Geometry: final body of the model. Coordinates: model frame, mm. A direction names the side the tool comes from. Give positions to 0.01 mm unless a question says otherwise; leave off trailing zeros. Write each loop counter-clockwise with the first axis right and the second up, starting at its lowest first coordinate (ties: lowest second). Pieces come first, ordered by that corner, then holes. Notation, with made-up numbers: (-3, -4) -> (14, -4) arc R23 cw to (14, 24) -> close; hole circle Ø2 at (60, 57.25). An arc over 180 degrees is marked (long way). Use CSV: the item, a comma, the result in double quotes. Start each with the question number.
1) Section D-D (y = 1). Count the separate pieces of the cut face and the enclosed holes in it, plus the area to 3 significant figures.
2) Material intervals for line 1 (Z direction, x = -110.72, y = 1.15); line 2 (Z direction, x = 65, y = 0.3); line 3 (X direction, y = 0.95, z = -155), sorted ascending. Write a range as [from, to].
3) Section A-A (x = 148). Output: boundary loops of the cut face in (y, z).
4) Set-up query: faces 1 (the face through (-2, 0, -2)), 2 (the face through (-62.018, 0.74, -149.464)). Return all of +Z, -Z, +X, -X, +Y, -Y with unobstructed straight access to the full face (end or side cutting, diameter ignored); none if empty.
5) Section B-B (z = 80). Output: boundary loops of the cut face in (x, y), plus the area to 3 significant figures.
6) Contact query for flat-ended pins moving along their axis: P1, Ø3, axis at x = 65, z = 118.58, coming from the -Y side; P2, Ø0.8, axis at x = -135.5, y = 1, coming from the -Z side. Output: stop coordinate, or through.
7) Draft query along X for faces 3 (the face through (-150, 1, -150)), 4 (the face through (150, 1, 150)), 5 (the face through (-1.35, 0.74, 122.74)). Return one class per face: pulls with the +X half, pulls with the -X half, needs draft (parallel to the pull), parting line crosses it, or undercut.
8) Section C-C (z = 148). Output: boundary loops of the cut face in (x, y).
```python
from build123d import *

# Parameters (mm, degrees)
SKETCH_1_R          = 1.55
SKETCH_1_W          = 30.4
SKETCH_1_H          = 68.58
EXTRUDE_1_DEPTH     = 1.5
FILLET_1_R          = 10
FILLET_2_R          = 10
FILLET_3_R          = 10
SKETCH_1_5_R        = 2.05
CUT_EXTRUDE_3_DEPTH = 10


with BuildPart() as part:
    # 草图1 → 凸台-拉伸1 (new body)
    with BuildSketch(Plane(origin=(0, 0, 0), x_dir=(1, 0, 0), z_dir=(0, 1, 0))):
        with BuildLine():
            Line((-125, 175), (-175, 125))
            Line((-175, 125), (-175, -125))
            Line((-175, -125), (-125, -175))
            Line((-125, -175), (-81.710313025, -175))
            ThreePointArc((-81.710313025, -175), (0, -122.728301649), (81.710313025, -175))
            Line((81.710313025, -175), (125, -175))
            Line((125, -175), (175, -125))
            Line((175, -125), (175, 125))
            Line((175, 125), (125, 175))
            Line((125, 175), (85, 175))
            Line((85, 175), (40, 125))
            Line((40, 125), (40, 85))
            Line((40, 85), (-40, 85))
            Line((-40, 85), (-40, 125))
            Line((-40, 125), (-85, 175))
            Line((-85, 175), (-125, 175))
        make_face()
        with Locations((-55, 131)):
            Circle(SKETCH_1_R, mode=Mode.SUBTRACT)
        with Locations((-80, 160)):
            Circle(SKETCH_1_R, mode=Mode.SUBTRACT)
        with Locations((55, 131)):
            Circle(SKETCH_1_R, mode=Mode.SUBTRACT)
        with Locations((80, 160)):
            Circle(SKETCH_1_R, mode=Mode.SUBTRACT)
        with Locations((-65, 118.58)):
            Circle(SKETCH_1_R, mode=Mode.SUBTRACT)
        with Locations((-65, 50)):
            Circle(SKETCH_1_R, mode=Mode.SUBTRACT)
        with Locations((-110.72, 50)):
            Circle(SKETCH_1_R, mode=Mode.SUBTRACT)
        with Locations((-110.72, 118.58)):
            Circle(SKETCH_1_R, mode=Mode.SUBTRACT)
        with Locations((-164.434, 118.58)):
            Circle(SKETCH_1_R, mode=Mode.SUBTRACT)
        with Locations((-164.434, 50)):
            Circle(SKETCH_1_R, mode=Mode.SUBTRACT)
        with Locations((-65, -118.58)):
            Circle(SKETCH_1_R, mode=Mode.SUBTRACT)
        with Locations((-65, -50)):
            Circle(SKETCH_1_R, mode=Mode.SUBTRACT)
        with Locations((-110.72, -50)):
            Circle(SKETCH_1_R, mode=Mode.SUBTRACT)
        with Locations((-110.72, -118.58)):
            Circle(SKETCH_1_R, mode=Mode.SUBTRACT)
        with Locations((-164.434, -50)):
            Circle(SKETCH_1_R, mode=Mode.SUBTRACT)
        with Locations((-164.434, -118.58)):
            Circle(SKETCH_1_R, mode=Mode.SUBTRACT)
        with Locations((65, 50)):
            Circle(SKETCH_1_R, mode=Mode.SUBTRACT)
        with Locations((110.72, 50)):
            Circle(SKETCH_1_R, mode=Mode.SUBTRACT)
        with Locations((110.72, 118.58)):
            Circle(SKETCH_1_R, mode=Mode.SUBTRACT)
        with Locations((65, 118.58)):
            Circle(SKETCH_1_R, mode=Mode.SUBTRACT)
        with Locations((164.434, 118.58)):
            Circle(SKETCH_1_R, mode=Mode.SUBTRACT)
        with Locations((164.434, 50)):
            Circle(SKETCH_1_R, mode=Mode.SUBTRACT)
        with Locations((164.434, -118.58)):
            Circle(SKETCH_1_R, mode=Mode.SUBTRACT)
        with Locations((164.434, -50)):
            Circle(SKETCH_1_R, mode=Mode.SUBTRACT)
        with Locations((110.72, -50)):
            Circle(SKETCH_1_R, mode=Mode.SUBTRACT)
        with Locations((110.72, -118.58)):
            Circle(SKETCH_1_R, mode=Mode.SUBTRACT)
        with Locations((65, -118.58)):
            Circle(SKETCH_1_R, mode=Mode.SUBTRACT)
        with Locations((65, -50)):
            Circle(SKETCH_1_R, mode=Mode.SUBTRACT)
        with Locations((-138.794, 84.29)):
            Rectangle(SKETCH_1_W, SKETCH_1_H, mode=Mode.SUBTRACT)
        with Locations((138.794, 84.29)):
            Rectangle(SKETCH_1_W, SKETCH_1_H, mode=Mode.SUBTRACT)
        with Locations((-138.794, -84.29)):
            Rectangle(SKETCH_1_W, SKETCH_1_H, mode=Mode.SUBTRACT)
        with Locations((138.794, -84.29)):
            Rectangle(SKETCH_1_W, SKETCH_1_H, mode=Mode.SUBTRACT)
    extrude(amount=EXTRUDE_1_DEPTH)

    # 圆角1
    fillet_1_edges = [part.edges().sort_by_distance(p)[0] for p in [
        (-40, 0.75, -125),
    ]]
    fillet(fillet_1_edges, radius=FILLET_1_R)

    # 圆角2
    fillet_2_edges = [part.edges().sort_by_distance(p)[0] for p in [
        (40, 0.75, -125),
    ]]
    fillet(fillet_2_edges, radius=FILLET_2_R)

    # 圆角3
    fillet_3_edges = [part.edges().sort_by_distance(p)[0] for p in [
        (175, 0.75, 125),
        (125, 0.75, 175),
        (81.710313025, 0.75, 175),
        (-81.710313025, 0.75, 175),
        (-125, 0.75, 175),
        (-175, 0.75, 125),
        (-175, 0.75, -125),
        (-125, 0.75, -175),
        (-85, 0.75, -175),
        (85, 0.75, -175),
        (125, 0.75, -175),
        (175, 0.75, -125),
    ]]
    fillet(fillet_3_edges, radius=FILLET_3_R)

    # 草图1<5> → 切除-拉伸3 (cut)
    with BuildSketch(Plane(origin=(0, 0, 0), x_dir=(1, 0, 0), z_dir=(0, 1, 0))):
        with Locations((90, 155)):
            Circle(SKETCH_1_5_R)
        with Locations((75, 155)):
            Circle(SKETCH_1_5_R)
        with Locations((90, 145)):
            Circle(SKETCH_1_5_R)
        with Locations((75, 145)):
            Circle(SKETCH_1_5_R)
        with Locations((-75, 145)):
            Circle(SKETCH_1_5_R)
        with Locations((-90, 155)):
            Circle(SKETCH_1_5_R)
        with Locations((-90, 145)):
            Circle(SKETCH_1_5_R)
        with Locations((-75, 155)):
            Circle(SKETCH_1_5_R)
    extrude(amount=CUT_EXTRUDE_3_DEPTH, mode=Mode.SUBTRACT)


solid = part.part
```
Answers follow:
1,separate pieces,"1"
1,enclosed holes,"40"
1,area,"93,200 mm^2"
2,line 1,"z = [-175, -120.13], [-117.03, -51.55], [-48.45, 48.45], [51.55, 117.03], [120.13, 175]"
2,line 2,"z = [-152.78, -120.13], [-117.03, -51.55], [-48.45, 48.45], [51.55, 117.03], [120.13, 150.48]"
2,line 3,"x = [-145, -92.05], [-87.95, -77.05], [-72.95, -67], [67, 72.95], [77.05, 87.95], [92.05, 145]"
3,outline,"(0, -152) -> (1.5, -152) -> (1.5, -118.58) -> (0, -118.58) -> close; (0, -50) -> (1.5, -50) -> (1.5, 50) -> (0, 50) -> close; (0, 118.58) -> (1.5, 118.58) -> (1.5, 152) -> (0, 152) -> close"
4,face 1,"+Z, -Z, +X, -X, -Y"
4,face 2,"-Z, +Y, -Y"
5,outline,"(-175, 0) -> (-153.99, 0) -> (-153.99, 1.5) -> (-175, 1.5) -> close; (-123.59, 0) -> (123.59, 0) -> (123.59, 1.5) -> (-123.59, 1.5) -> close; (153.99, 0) -> (175, 0) -> (175, 1.5) -> (153.99, 1.5) -> close"
5,area,"434 mm^2"
6,P1,"passes through"
6,P2,"stops at z = -164.9"
7,face 3,"pulls with the -X half"
7,face 4,"pulls with the +X half"
7,face 5,"undercut"
8,outline,"(-152, 0) -> (-62.53, 0) -> (-62.53, 1.5) -> (-152, 1.5) -> close; (62.53, 0) -> (152, 0) -> (152, 1.5) -> (62.53, 1.5) -> close"
